```python
from build123d import *

# Parameters (mm, degrees)
F1_DEPTH = 25.4
F2_T     = -3.175


with BuildPart() as f1:
    # F0 (on Top) → F1 (new body)
    with BuildSketch(Plane.XY):
        with BuildLine():
            Line((-133.35, 86.135591), (-133.35, -86.135591))
            ThreePointArc((-133.35, -86.135591), (0, -158.75), (133.35, -86.135591))
            Line((133.35, -86.135591), (133.35, 86.135591))
            ThreePointArc((133.35, 86.135591), (0, 158.75), (-133.35, 86.135591))
        make_face()
    extrude(amount=-F1_DEPTH)

    # F2
    f2_openings = [f1.faces().sort_by_distance(p)[0] for p in [
        (0, 0, 0),
    ]]
    offset(amount=F2_T, openings=f2_openings)


solid = f1.part
```
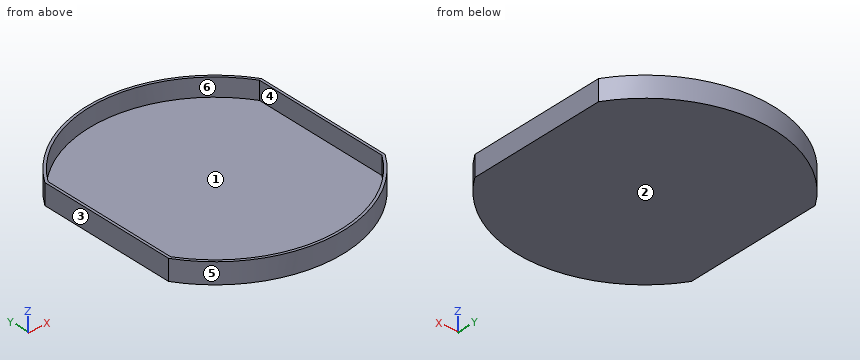
Check sheet for the modelled part. Datum: model origin and axes. Units: mm. Face numbers are marked on the shaded views. A direction names the side the tool comes from. Round coordinates to 2 decimals unless told otherwise and drop trailing zeros. Loops run counter-clockwise (first coordinate to the right, second up) from the corner with the lowest first, then second, coordinate; pieces in that order, holes last. Notation, with made-up numbers: (59.5, 41) -> (73.5, 41) arc R12 cw to (73.5, 58) -> close; hole circle Ø10 at (24.25, -12.5). An arc over 180 degrees is marked (long way). Answer in a Markdown table with one row per item.
Q1. Set-up check for the marked faces 1 and 2: record each of +Z, -Z, +X, -X, +Y, -Y from which the full face is reachable in a straight line by a thin tool's end or side.
Data:
| item | result |
|---|---|
| face 1 | +Z |
| face 2 | -Z, +X, -X, +Y, -Y |
Q2. Sectioned sample at C-C on x = -22. Enter the section's corners in (y, z) (3 decimals), then the cut area to 3 significant figures.
Data:
| item | result |
|---|---|
| outline | (-157.218, -25.4) -> (157.218, -25.4) -> (157.218, 0) -> (154.012, 0) -> (154.012, -22.225) -> (-154.012, -22.225) -> (-154.012, 0) -> (-157.218, 0) -> close |
| area | 1,140 mm^2 |
Q3. Sectioned sample at A-A on z = -9.5. Enter the section's corners in (x, y) (3 decimals), then the cut area to 3 significant figures.
Data:
| item | result |
|---|---|
| outline | (-133.35, -86.136) arc R158.75 ccw to (133.35, -86.136) -> (133.35, 86.136) arc R158.75 ccw to (-133.35, 86.136) -> close; hole (-130.175, -85.194) arc R155.575 ccw to (130.175, -85.194) -> (130.175, 85.194) arc R155.575 ccw to (-130.175, 85.194) -> close |
| area | 3,070 mm^2 |
Q4. Thickness scan on L1, parallel to X at y = 60.5, z = -17.5 (3 decimals); L2, parallel to Y at x = 3, z = -18.25; L3, parallel to Z at x = -37, y = 22.5 (3 decimals). Record the ranges inside material, lowest first.
Data:
| item | result |
|---|---|
| L1 | x = -133.35 to -130.175, 130.175 to 133.35 |
| L2 | y = -158.72 to -155.55, 155.55 to 158.72 |
| L3 | z = -25.4 to -22.225 |
Q5. Release check for a two-part mould opening along X. For the marked faces 3, 4, 5 and 6 record: released by +X, released by -X, zero draft, split by the parting line, or undercut.
Data:
| item | result |
|---|---|
| face 3 | released by -X |
| face 4 | undercut |
| face 5 | split by the parting line |
| face 6 | undercut |
Q6. Sectioned sample at B-B on y = 17. Enter the section's corners in (x, z) (3 decimals).
Data:
| item | result |
|---|---|
| outline | (-133.35, -25.4) -> (133.35, -25.4) -> (133.35, 0) -> (130.175, 0) -> (130.175, -22.225) -> (-130.175, -22.225) -> (-130.175, 0) -> (-133.35, 0) -> close |
Q7. Go/stop test with flat-tipped pins: P1, Ø10, axis at x = 90, z = -9, coming from the +Y side; P2, Ø8, axis at x = 37.5, z = -18, coming from the -Y side; P3, Ø4, axis at x = -71, z = -3, coming from the +Y side. Record where each tip stops, or that it passes through.
Data:
| item | result |
|---|---|
| P1 | stops at y = 134.08 |
| P2 | stops at y = -155.18 |
| P3 | stops at y = 142.97 |
